The listing builds one solid part. Answer for the finished solid, in the listing's coordinates (mm). Give positions to 0.01 mm unless a question says otherwise; leave off trailing zeros. Loops run counter-clockwise (first coordinate to the right, second up) from the corner with the lowest first, then second, coordinate; pieces in that order, holes last. Notation, with made-up numbers: (66, 21) - (81, 21) arc R14 ccw to (81, 36) - close; hole circle Ø6 at (55, 56.5). An arc over 180 degrees is marked (long way). Write each question's results on one line, items separated by ' | '.
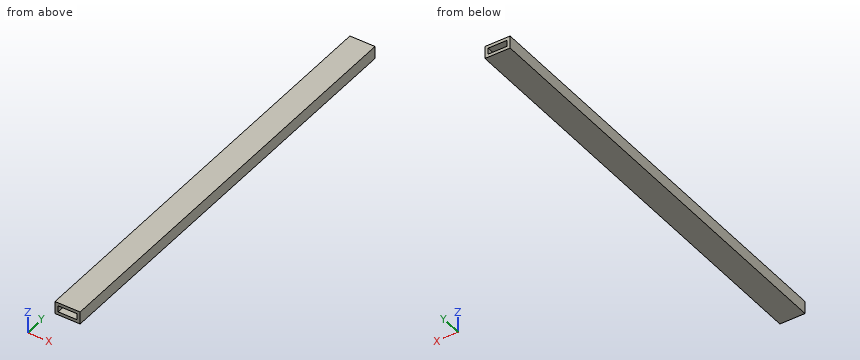
from build123d import *

# Parameters (mm, degrees)
F0_W     = 19.05
F0_H     = 6.35
F1_DEPTH = 265.43
F2_W     = 25.4
F2_H     = 12.7
F2_W_2   = 19.05
F2_H_2   = 6.35
F3_DEPTH = 86.36
F4_DEPTH = 86.36


with BuildPart() as f1:
    # F0 (on Front) → F1 (new body)
    with BuildSketch(Plane.XZ):
        Polygon((-25.4, 0), (0, 0), (0, 12.7), (-25.4, 12.7), (-25.4, 9.525), align=None)
        with Locations((-12.7, 6.35)):
            Rectangle(F0_W, F0_H, mode=Mode.SUBTRACT)
    extrude(amount=F1_DEPTH)

    # F2 (on face) → F3 (join)
    with BuildSketch(Plane.XZ.offset(265.43)):
        with Locations((-12.7, 6.35)):
            Rectangle(F2_W, F2_H)
        with Locations((-12.7, 6.35)):
            Rectangle(F2_W_2, F2_H_2, mode=Mode.SUBTRACT)
    extrude(amount=F3_DEPTH)

    # F4 (add): a face of the model
    f4_faces = [f1.faces().sort_by_distance(p)[0] for p in [
        (-12.7, 0, 0.2839806331),
    ]]
    extrude(f4_faces, amount=F4_DEPTH)


solid = f1.part
Item 1: A cutting plane is placed at B-B, the plane z = 7.5. Determine the outline of the cut face in (x, y) (3 decimals).
Values found:
outline: (-25.4, -351.79) - (-22.225, -351.79) - (-22.225, 86.36) - (-25.4, 86.36) - close; (-3.175, -351.79) - (0, -351.79) - (0, 86.36) - (-3.175, 86.36) - close
Item 2: A cutting plane is placed at A-A, the plane x = -9.5. Determine the outline of the cut face in (y, z) (3 decimals).
Values found:
outline: (-351.79, 0) - (86.36, 0) - (86.36, 3.175) - (-351.79, 3.175) - close; (-351.79, 9.525) - (86.36, 9.525) - (86.36, 12.7) - (-351.79, 12.7) - close
Item 3: A cutting plane is placed at C-C, the plane y = -136.5. Determine the outline of the cut face in (x, z) (3 decimals).
Values found:
outline: (-25.4, 0) - (0, 0) - (0, 12.7) - (-25.4, 12.7) - close; hole (-22.225, 3.175) - (-3.175, 3.175) - (-3.175, 9.525) - (-22.225, 9.525) - close
Item 4: Find the intervals of material crossed by line 1 along X through (y, z) = (-25.5, 5.25) (3 decimals); line 2 along Z through (x, y) = (-20.5, -49) (3 decimals), in increasing order. Write a range as [from, to].
Values found:
line 1: x = [-25.4, -22.225], [-3.175, 0] | line 2: z = [0, 3.175], [9.525, 12.7]
